```python
from build123d import *

# Parameters (mm, degrees)
SKETCH_1_R        = 2.5
EXTRUDE_198_DEPTH = 30
SKETCH_6_W        = 4.5
SKETCH_6_H        = 1
PH2_START         = 1.01
PH2_DEPTH         = 0.66


with BuildPart() as part:
    # 草图1 → Extrude 198 (new body)
    with BuildSketch(Plane.XY):
        Circle(SKETCH_1_R)
    extrude(amount=-EXTRUDE_198_DEPTH)

    # 草图6 → Revolve 324 (revolve)
    with BuildSketch(Plane(origin=(0, 0, 0), x_dir=(1, 0, 0), z_dir=(0, 1, 0)), mode=Mode.PRIVATE) as revolve_324_sk:
        with Locations((2.25, -0.5)):
            Rectangle(SKETCH_6_W, SKETCH_6_H)
    revolve(revolve_324_sk.sketch.rotate(Axis((0, 0, -2), (0, 0, 1)), 180), axis=Axis((0, 0, -2), (0, 0, 1)))

    # 草图7 → 十字槽_PH2_简化 (cut)
    with BuildSketch(Plane.XY.offset(PH2_START)):
        Polygon((-0.45, -1.5), (0.45, -1.5), (0.45, -0.45), (1.5, -0.45), (1.5, 0.45), (0.45, 0.45), (0.45, 1.5), (-0.45, 1.5), (-0.45, 0.45), (-1.5, 0.45), (-1.5, -0.45), (-0.45, -0.45), align=None)
    extrude(amount=-PH2_DEPTH, mode=Mode.SUBTRACT)


solid = part.part
```
Read the model definition and answer for the solid it produces. Units are mm, in the model's axes. A direction names the side the tool comes from. Coordinates: 2 decimals unless noted, no trailing zeros. Order: outer loops, then holes, each group sorted by start corner. A loop starts at its lowest first (then second) coordinate and runs counter-clockwise, first axis right, second up. Notation, with made-up numbers: (87.5, -26.75) - (118.5, -26.75) arc R29 ccw to (118.5, -1.75) - close; hole circle Ø3 at (79.25, 46). An arc over 180 degrees is marked (long way). Answer as a JSON object with one key per item and string values. Group by question number.
Item 1: Section D-D (y = 3) is taken. Give the vertices of the cut face in (x, z).
Item 2: The mould has two halves that part along Y. Classify faces 1 (the face through (3.32, -3.04, 0.49)), 2 (the face through (2, 2, 0)), 3 (the face through (0, 0, 0.35)): +Y half, -Y half, draft (parallel to the pull), parting line (faces both ways), or undercut.
Item 3: A tool of negligible diameter and unlimited length cuts with its end or side. For faces 4 (the face through (-0.54, -2.44, -14.79)), 5 (the face through (0, 0, -30)), from which of +Z, -Z, +X, -X, +Y, -Y can it reach the whole face along a straight path? Write none if from no direction.
Item 4: Section C-C (z = -6.5) is taken. Give the vertices of the cut face in (x, y), plus the area to 3 significant figures.
Item 5: Section A-A (y = 0) is taken. Give the vertices of the cut face in (x, z).
Item 6: Flat-ended cylindrical pins translate along their axes: P1, Ø0.5, axis at y = 1, z = 0.5, coming from the -X side; P2, Ø0.7, axis at y = 1, z = 0.5, coming from the +X side; P3, Ø0.7, axis at x = -1, z = 1, coming from the -Y side; P4, Ø2.5, axis at x = 0, y = 0, coming from the +Z side. Find the tip coordinate at first contact, or state that the pin passes through.
Item 7: Consider probe 1 along Y at (x, z) = (2, -26); probe 2 along Z at (x, y) = (0.5, 3.25); probe 3 along Y at (x, z) = (0.75, -24.5). Determine where each line is inside the solid, lowest interval first. Write a range as from..to.
Results are:
{
 "1": {"outline": "(-3.35, 0) - (3.35, 0) - (3.35, 1) - (-3.35, 1) - close"},
 "2": {"face 1": "parting line", "face 2": "draft", "face 3": "undercut"},
 "3": {"face 4": "-Z", "face 5": "-Z, +X, -X, +Y, -Y"},
 "4": {"outline": "circle Ø5 at (0, 0)", "area": "19.6 mm^2"},
 "5": {"outline": "(-4.5, 0) - (-2.5, 0) - (-2.5, -30) - (2.5, -30) - (2.5, 0) - (4.5, 0) - (4.5, 1) - (1.5, 1) - (1.5, 0.35) - (-1.5, 0.35) - (-1.5, 1) - (-4.5, 1) - close"},
 "6": {"P1": "stops at x = -4.44", "P2": "stops at x = 4.45", "P3": "stops at y = -4.45", "P4": "stops at z = 1"},
 "7": {"probe 1": "y = -1.5..1.5", "probe 2": "z = 0..1", "probe 3": "y = -2.38..2.38"}
}
